Check sheet for the modelled part. Datum: model origin and axes. Units: mm. Round coordinates to 2 decimals unless told otherwise and drop trailing zeros. Write each loop counter-clockwise with the first axis right and the second up, starting at its lowest first coordinate (ties: lowest second). Pieces come first, ordered by that corner, then holes. Notation, with made-up numbers: M 60,61 L 76,61 A7 cw 76,69 Z; hole C -17.5,-6 d4. An arc over 180 degrees is marked long. Put each result on its own line as item: value.
Autodesk Inventor part; units mm, degrees
ref_plane "YZ Plane" through (0, 0, 0) normal (1, 0, 0) x (0, 1, 0)
ref_plane "XZ Plane" through (0, 0, 0) normal (0, 1, 0) x (-1, 0, 0)
ref_plane "XY Plane" through (0, 0, 0) normal (0, 0, 1) x (1, 0, 0)
sketch "草圖1" plane through (0, 0, 0) normal (0, 0, 1) x (1, 0, 0)
  circle A0 centre (15, 0) radius 1.5
  circle A1 centre (-7.5, -12.9904) radius 1.5
  circle A2 centre (-7.5, 12.9904) radius 1.5
  circle A3 centre (0, 0) radius 9.94
  arc A4 (24.2558, 6.0545) -> (-24.6882, 3.9362) centre (0, 0) ccw
  arc A5 (-25.4732, -69.9345) -> (3.0268, -98.4345) centre (3.0268, -69.9345) ccw
  arc A6 (3.0268, -98.4345) -> (31.5268, -69.9345) centre (3.0268, -69.9345) ccw
  arc A7 (-35.4868, -63.7941) -> (40.8658, -60.4896) centre (3.0268, -69.9345) ccw
  line L0 (24.2558, 6.0545) -> (40.8658, -60.4896)
  line L1 (-24.6882, 3.9362) -> (-35.4868, -63.7941)
  circle A8 centre (26.5268, -93.4345) radius 2.5
  circle A9 centre (-20.4732, -93.4345) radius 2.5
  circle A10 centre (-20.4732, -46.4345) radius 2.5
  circle A11 centre (26.5268, -46.4345) radius 2.5
  circle A12 centre (3.0268, -69.9345) radius 19
  circle A13 centre (3.0268, -69.9345) radius 19.5
  circle A14 centre (0, 0) radius 10.5
  point P0 (0, 0)
  dimension "d1" = 50
  dimension "d2" = 78
  dimension "d3" = 39
  dimension "d4" = 21
extrude "擠出1" add sketch "草圖1" along normal blind 4 contours L0 A7 L1 A4
properties part number "Linker_Structure"
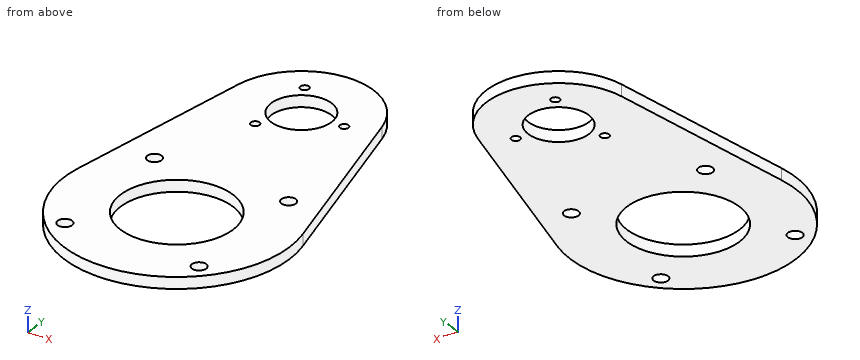
1. Depth check by flat-ended pin: pin 1 Ø4.5 at (x, y) = (-20.47, -46.43) entering from -Z. Enter the tip coordinate at first touch or a pass-through.
Computed values:
pin 1: passes through
2. Cross-section at B-B (x = 15). Enter the section's corners in (y, z), then the cut area to 3 significant figures.
Computed values:
outline: M -107.05,0 L -85.33,0 L -85.33,4 L -107.05,4 Z; M -54.54,0 L -1.5,0 L -1.5,4 L -54.54,4 Z; M 1.5,0 L 20,0 L 20,4 L 1.5,4 Z
area: 373 mm2
3. Cross-section at D-D (x = -7.5). Enter the section's corners in (y, z).
Computed values:
outline: M -107.49,0 L -86.35,0 L -86.35,4 L -107.49,4 Z; M -53.52,0 L -14.49,0 L -14.49,4 L -53.52,4 Z; M -11.49,0 L -7.35,0 L -7.35,4 L -11.49,4 Z; M 7.35,0 L 11.49,0 L 11.49,4 L 7.35,4 Z; M 14.49,0 L 23.85,0 L 23.85,4 L 14.49,4 Z
4. Scan lines: probe 1 along Y at (x, z) = (8, 2.55); probe 2 along X at (y, z) = (-45.5, 0.2); probe 3 along X at (y, z) = (-46.5, 2.6). Record each from-to range of solid material in increasing order.
Computed values:
probe 1: y = -108.62 to -88.79, -51.08 to -6.8, 6.8 to 23.69
probe 2: x = -32.57 to -22.79, -18.15 to 24.21, 28.85 to 37.12
probe 3: x = -32.73 to -22.97, -17.97 to 24.03, 29.03 to 37.37
5. Cross-section at C-C (z = 1.6). Count the separate pieces of the cut face and the enclosed holes in it, then the cut area to 3 significant figures.
Computed values:
separate pieces: 1
enclosed holes: 9
area: 6,300 mm2
6. Cross-section at A-A (y = -78). Enter the section's corners in (x, z), then the cut area to 3 significant figures.
Computed values:
outline: M -35.13,0 L -14.73,0 L -14.73,4 L -35.13,4 Z; M 20.78,0 L 41.18,0 L 41.18,4 L 20.78,4 Z
area: 163 mm2
